Input: part model. Units: mm. Frame: model coordinates. A direction names the side the tool comes from. Give positions to 0.01 mm unless a question says otherwise; leave off trailing zeros. Loops run counter-clockwise (first coordinate to the right, second up) from the corner with the lowest first, then second, coordinate; pieces in that order, holes last.
from build123d import *

# Parameters (mm, degrees)
F0_W     = 190.5
F0_H     = 127
F1_DEPTH = 11.176
F3_D     = 14.2875
F4_W     = 92.075
F4_H     = 6.35
F4_W_2   = 6.35
F4_H_2   = 60.325
F5_DEPTH = 152.4
F6_W     = 190.5
F6_H     = 127
F7_DEPTH = 11.176
F9_DEPTH = 25.4


# Not quite as in the source:
# - a length typed as a fraction of an inch, garbled in the dataset ("3 / 203.2 mm" for 3/8 in), is restored


with BuildPart() as f1:
    # F0 (on Top) → F1 (new body)
    with BuildSketch(Plane.XY):
        Rectangle(F0_W, F0_H)
    extrude(amount=F1_DEPTH)

    # F3 (through all)
    with Locations(Plane.XY.offset(11.176)):
        with Locations((-79.375, 47.625), (79.375, 47.625), (-79.375, -47.625), (79.375, -47.625)):
            Hole(F3_D / 2)

    # F4 (on face) → F5 (join)
    with BuildSketch(Plane.XY.offset(11.176)):
        with Locations((-49.2125, 0)):
            Rectangle(F4_W, F4_H)
        with Locations((0, 33.3375)):
            Rectangle(F4_W_2, F4_H_2)
        Rectangle(F4_W_2, F4_H)
        with Locations((49.2125, 0)):
            Rectangle(F4_W, F4_H)
        with Locations((0, -33.3375)):
            Rectangle(F4_W_2, F4_H_2)
    extrude(amount=F5_DEPTH)

    # F6 (on face) → F7 (join)
    with BuildSketch(Plane.XY.offset(163.576)):
        Rectangle(F6_W, F6_H)
    extrude(amount=F7_DEPTH)

    # F8 (on face) → F9 (cut)
    with BuildSketch(Plane.XY.offset(174.752)):
        with BuildLine():
            ThreePointArc((-69.088, -45.974), (-63.5, -51.562), (-57.912, -45.974))
            Line((-57.912, -45.974), (-57.912, -30.099))
            ThreePointArc((-57.912, -30.099), (-63.5, -24.511), (-69.088, -30.099))
            Line((-69.088, -30.099), (-69.088, -45.974))
        make_face()
        with BuildLine():
            Line((-57.912, 30.099), (-57.912, 45.974))
            ThreePointArc((-57.912, 45.974), (-63.5, 51.562), (-69.088, 45.974))
            Line((-69.088, 45.974), (-69.088, 30.099))
            ThreePointArc((-69.088, 30.099), (-63.5, 24.511), (-57.912, 30.099))
        make_face()
        with BuildLine():
            Line((69.088, 30.099), (69.088, 45.974))
            ThreePointArc((69.088, 45.974), (63.5, 51.562), (57.912, 45.974))
            Line((57.912, 45.974), (57.912, 30.099))
            ThreePointArc((57.912, 30.099), (63.5, 24.511), (69.088, 30.099))
        make_face()
        with BuildLine():
            Line((57.912, -30.099), (57.912, -45.974))
            ThreePointArc((57.912, -45.974), (63.5, -51.562), (69.088, -45.974))
            Line((69.088, -45.974), (69.088, -30.099))
            ThreePointArc((69.088, -30.099), (63.5, -24.511), (57.912, -30.099))
        make_face()
    extrude(amount=-F9_DEPTH, mode=Mode.SUBTRACT)


solid = f1.part
(1) Ray query, probe 1 along Z at (x, y) = (28, 45); probe 2 along Y at (x, z) = (-34.5, 76) (3 decimals). Return the intervals inside material, ascending.
Values follow:
probe 1: z = 0 to 11.18, 163.58 to 174.75
probe 2: y = -3.175 to 3.175
(2) Pin query (flat end, axial travel): pin 1 Ø2 at (y, z) = (-44, 117.5) entering from +X (3 decimals); pin 2 Ø4 at (y, z) = (-25.5, 94) entering from -X (3 decimals); pin 3 Ø3 at (x, z) = (16.5, 91.5) entering from +Y (3 decimals). Return the tip coordinate at first contact, or that it passes through.
Values follow:
pin 1: stops at x = 3.175
pin 2: stops at x = -3.175
pin 3: stops at y = 3.175
(3) Cut plane D-D (x = -33.5). Return the cut outline in (y, z) (3 decimals), and give its area (3 significant figures).
Values follow:
outline: (-63.5, 0) - (63.5, 0) - (63.5, 11.176) - (3.175, 11.176) - (3.175, 163.576) - (63.5, 163.576) - (63.5, 174.752) - (-63.5, 174.752) - (-63.5, 163.576) - (-3.175, 163.576) - (-3.175, 11.176) - (-63.5, 11.176) - close
area: 3,810 mm2
(4) Cut plane A-A (x = -63.5). Return the cut outline in (y, z) (3 decimals).
Values follow:
outline: (-63.5, 0) - (63.5, 0) - (63.5, 11.176) - (3.175, 11.176) - (3.175, 163.576) - (24.511, 163.576) - (24.511, 174.752) - (-24.511, 174.752) - (-24.511, 163.576) - (-3.175, 163.576) - (-3.175, 11.176) - (-63.5, 11.176) - close; (-63.5, 163.576) - (-51.562, 163.576) - (-51.562, 174.752) - (-63.5, 174.752) - close; (51.562, 163.576) - (63.5, 163.576) - (63.5, 174.752) - (51.562, 174.752) - close
(5) Reachability of faces 4 (the cylindrical face through (-74.11, 52.453, 5.51)), 5 (the flat face through (-50, 3.175, 86)), 6 (the flat face through (-50, -33, 163.576)), 7 (the flat face through (-69.088, -38, 169)), 8 (the flat face through (49, -33, 163.576)) from +Z, -Z, +X, -X, +Y, -Y: full face, straight path, thin tool, end or side. Return the list, or none.
Values follow:
face 4: -Z
face 5: -X, +Y
face 6: -X, -Y
face 7: +Z
face 8: +X, -Y
(6) Mould query, pull axis Z, two halves, no side actions, for faces 1 (the flat face through (69.088, 38, 169)), 2 (the flat face through (-1, 1, 174.752)), 3 (the flat face through (-50, 34, 163.576)). Classes: +Z half, -Z half, draft (parallel to the pull), parting line (faces both ways), or undercut.
Values follow:
face 1: draft
face 2: +Z half
face 3: undercut
(7) Cut plane B-B (z = 142.5). Return the cut outline in (x, y) (3 decimals), and give its area (3 significant figures).
Values follow:
outline: (-95.25, -3.175) - (-3.175, -3.175) - (-3.175, -63.5) - (3.175, -63.5) - (3.175, -3.175) - (95.25, -3.175) - (95.25, 3.175) - (3.175, 3.175) - (3.175, 63.5) - (-3.175, 63.5) - (-3.175, 3.175) - (-95.25, 3.175) - close
area: 1,980 mm2
(8) Cut plane C-C (y = -27.5). Return the cut outline in (x, z) (3 decimals), and give its area (3 significant figures).
Values follow:
outline: (-95.25, 0) - (95.25, 0) - (95.25, 11.176) - (3.175, 11.176) - (3.175, 163.576) - (58.553, 163.576) - (58.553, 174.752) - (-58.553, 174.752) - (-58.553, 163.576) - (-3.175, 163.576) - (-3.175, 11.176) - (-95.25, 11.176) - close; (-95.25, 163.576) - (-68.447, 163.576) - (-68.447, 174.752) - (-95.25, 174.752) - close; (68.447, 163.576) - (95.25, 163.576) - (95.25, 174.752) - (68.447, 174.752) - close
area: 5,000 mm2
